Work out the finished part from the listing and answer in its coordinate system (mm). A direction names the side the tool comes from. Give positions to 0.01 mm unless a question says otherwise; leave off trailing zeros. Order: outer loops, then holes, each group sorted by start corner. A loop starts at its lowest first (then second) coordinate and runs counter-clockwise, first axis right, second up.
```python
from build123d import *

# Parameters (mm, degrees)
F2_R     = 5
F3_R     = 25
F4_DEPTH = 10


with BuildPart() as f1:
    # F0 (on Front) → F1 (revolve)
    with BuildSketch(Plane.XZ):
        Polygon((-60.746692, 14), (-60.746692, 0), (-45, 0), (-45, -33), (-21.65, -33), (-21.65, 37), (-45, 37), (-45, 14), align=None)
    revolve(axis=Axis((0, 0, 28.312229), (0, 0, 1)))

    # F2
    f2_edges = [f1.edges().sort_by_distance(p)[0] for p in [
        (45, 0, 37),
    ]]
    fillet(f2_edges, radius=F2_R)

    # F3 (on face) → F4 (cut)
    with BuildSketch(Plane(origin=(0, 0, -33), x_dir=(1, 0, 0), z_dir=(0, 0, -1))):
        Circle(F3_R)
    extrude(amount=-F4_DEPTH, mode=Mode.SUBTRACT)


solid = f1.part
```
1. Which of the six approach directions +Z, -Z, +X, -X, +Y, -Y give full straight-line access (tool end or side, diameter ignored) to faces 1 (the face through (-45.3, -0.3, 14)), 2 (the face through (45.3, -0.3, 0)), 3 (the face through (-57.94, -18.25, 6.9))?
Findings below:
face 1: +Z
face 2: -Z
face 3: +Z, -Z
2. Given P1, Ø1, axis at y = 42, z = -9.5, coming from the -X side; P2, Ø8, axis at x = -43, y = -24.5, coming from the -Z side; P3, Ø3, axis at y = -21.5, z = -15, coming from the -X side, each flat-ended and moving along its own axis, determine where each tip first touches the part or whether it passes through.
Findings below:
P1: stops at x = -17.4
P2: stops at z = 0
P3: stops at x = -40.31
3. Straight lines are drawn through the part: probe 1 along X at (y, z) = (0, -2.5); probe 2 along Y at (x, z) = (0, 9); probe 3 along Y at (x, z) = (0, -28.5). For each, find the intervals that lie inside material, in ascending order.
Findings below:
probe 1: x = -45 to -21.65, 21.65 to 45
probe 2: y = -60.75 to -21.65, 21.65 to 60.75
probe 3: y = -45 to -25, 25 to 45
4. The part is cut by section C-C (z = 22). Write down the section's boundary in (x, y).
Findings below:
outline: circle Ø90 at (0, 0); hole circle Ø43.3 at (0, 0)
5. The mould has two halves that part along X. Classify faces 4 (the face through (-20.765, 39.923, 22.874)), 5 (the face through (17, 17, 37)), 6 (the face through (23.846, -7.509, -28.07)): pulls with the +X half, pulls with the -X half, needs draft (parallel to the pull), parting line crosses it, or undercut.
Findings below:
face 4: parting line crosses it
face 5: needs draft
face 6: undercut
6. The part is cut by section A-A (y = 0). Write down the section's boundary in (x, z), then the cut area to 3 significant figures.
Findings below:
outline: (-60.75, 0) - (-45, 0) - (-45, -33) - (-25, -33) - (-25, -23) - (-21.65, -23) - (-21.65, 37) - (-40, 37) arc R5 ccw to (-45, 32) - (-45, 14) - (-60.75, 14) - close; (21.65, -23) - (25, -23) - (25, -33) - (45, -33) - (45, 0) - (60.75, 0) - (60.75, 14) - (45, 14) - (45, 32) arc R5 ccw to (40, 37) - (21.65, 37) - close
area: 3,630 mm2
7. The part is cut by section D-D (y = -52.5). Write down the section's boundary in (x, z).
Findings below:
outline: (-30.56, 0) - (30.56, 0) - (30.56, 14) - (-30.56, 14) - close
